Source: CAD feature listing. Evaluate the final solid. Frame: model axes, mm. A direction names the side the tool comes from. Give positions to 0.01 mm unless a question says otherwise; leave off trailing zeros. Loops run counter-clockwise (first coordinate to the right, second up) from the corner with the lowest first, then second, coordinate; pieces in that order, holes last.
Autodesk Inventor part; units mm, degrees
ref_plane "YZ Plane" through (0, 0, 0) normal (1, 0, 0) x (0, 1, 0)
ref_plane "XZ Plane" through (0, 0, 0) normal (0, 1, 0) x (-1, 0, 0)
ref_plane "XY Plane" through (0, 0, 0) normal (0, 0, 1) x (1, 0, 0)
sketch "Sketch1" plane through (0, 0, 0) normal (0, 1, 0) x (-1, 0, 0)
  circle A0 centre (0, 0) radius 55
  dimension "d0" = 110
extrude "Extrusion1" add sketch "Sketch1" along normal blind 40
sketch "Sketch2" plane through (0, 0, 0) normal (0, -1, 0) x (1, 0, 0)
  circle A0 centre (0, 0) radius 44
  circle A1 centre (0, 0) radius 55
  dimension "d3" = 88
extrude "Extrusion2" cut sketch "Sketch2" against normal blind 36
sketch "Sketch3" plane through (0, 40, 0) normal (0, 1, 0) x (1, 0, 0)
  circle A0 centre (0, 0) radius 30
  dimension "d6" = 60
extrude "Extrusion3" cut sketch "Sketch3" against normal through all
sketch "Sketch4" plane through (0, 40, 0) normal (0, 1, 0) x (1, 0, 0)
  circle A0 centre (0, 0) radius 40
  dimension "d9" = 80
extrude "Extrusion4" cut sketch "Sketch4" against normal blind 36
sketch "Sketch5" plane through (0, 40, 0) normal (0, 1, 0) x (1, 0, 0)
  circle A0 centre (0, 0) radius 47.5
  circle A1 centre (0, 47.5) radius 2
  circle A2 centre (-47.5, 0) radius 2
  circle A3 centre (0, -47.5) radius 2
  circle A4 centre (47.5, 0) radius 2
  dimension "d12" = 95
  dimension "d13" = 4
  dimension "d16" = 360
hole "Hole1" at (-47.5, 40, 0) at (0, 40, 47.5) at (47.5, 40, 0) at (0, 40, -47.5) direction (0, -1, 0) diameter 3 end through all
thread "Thread1"
thread "Thread2"
thread "Thread3"
thread "Thread4"
properties part number "sensor1_lock" material "Aluminum 6061"
1) Pull-direction query (Z, two-part tool) for faces 4 (the flat face through (-29, 0, -9)), 5 (the cylindrical face through (-9.538, 17.748, -42.954)), 6 (the cylindrical face through (0, 38, 46)); classes: released by +Z, released by -Z, zero draft, split by the parting line, or undercut.
Checks:
face 4: zero draft
face 5: split by the parting line
face 6: undercut
2) Contact query for flat-ended pins moving along their axis: P1, Ø12, axis at y = 13, z = -37, coming from the +X side (3 decimals); P2, Ø2.5, axis at x = 47.5, z = 0, coming from the -Y side; P3, Ø3, axis at x = 2, y = 5, coming from the +Z side; P4, Ø12, axis at y = 20, z = 15, coming from the +X side. Output: stop coordinate, or through.
Checks:
P1: stops at x = 31.225
P2: passes through
P3: stops at z = 44
P4: stops at x = 43.07
3) Cut plane D-D (z = 47.5). Return loops of the section in (x, y), and give its area (3 significant figures).
Checks:
outline: (-27.73, 36) - (-1.5, 36) - (-1.5, 40) - (-27.73, 40) - close; (1.5, 36) - (27.73, 36) - (27.73, 40) - (1.5, 40) - close
area: 210 mm2
4) Ray query, probe 1 along Z at (x, y) = (0, 2.85); probe 2 along Z at (x, y) = (-47.5, 38.75); probe 3 along Y at (x, z) = (-41.5, -15). Return the intervals inside material, ascending.
Checks:
probe 1: z = -44 to -30, 30 to 44
probe 2: z = -27.73 to -1.5, 1.5 to 27.73
probe 3: y = 36 to 40
5) Cut plane A-A (z = 0). Return loops of the section in (x, y).
Checks:
outline: (-55, 36) - (-49, 36) - (-49, 40) - (-55, 40) - close; (-46, 36) - (-44, 36) - (-44, 0) - (-30, 0) - (-30, 4) - (-40, 4) - (-40, 40) - (-46, 40) - close; (30, 0) - (44, 0) - (44, 36) - (46, 36) - (46, 40) - (40, 40) - (40, 4) - (30, 4) - close; (49, 36) - (55, 36) - (55, 40) - (49, 40) - close
6) Cut plane B-B (x = 0). Return loops of the section in (y, z).
Checks:
outline: (0, -44) - (36, -44) - (36, -46) - (40, -46) - (40, -40) - (4, -40) - (4, -30) - (0, -30) - close; (0, 30) - (4, 30) - (4, 40) - (40, 40) - (40, 46) - (36, 46) - (36, 44) - (0, 44) - close; (36, -55) - (40, -55) - (40, -49) - (36, -49) - close; (36, 49) - (40, 49) - (40, 55) - (36, 55) - close
7) Cut plane C-C (x = 18). Return loops of the section in (y, z), and give its area (3 significant figures).
Checks:
outline: (0, -40.15) - (36, -40.15) - (36, -51.97) - (40, -51.97) - (40, -35.72) - (4, -35.72) - (4, -24) - (0, -24) - close; (0, 24) - (4, 24) - (4, 35.72) - (40, 35.72) - (40, 51.97) - (36, 51.97) - (36, 40.15) - (0, 40.15) - close
area: 543 mm2
8) Reachability of faces 1 (the cylindrical face through (-8.67, 22.25, 39.05)), 2 (the cylindrical face through (11.923, 37.972, 53.692)), 3 (the flat face through (-17, 36, 41)) from +Z, -Z, +X, -X, +Y, -Y: full face, straight path, thin tool, end or side. Return the list, or none.
Checks:
face 1: +Y
face 2: +Y, -Y
face 3: -Y
